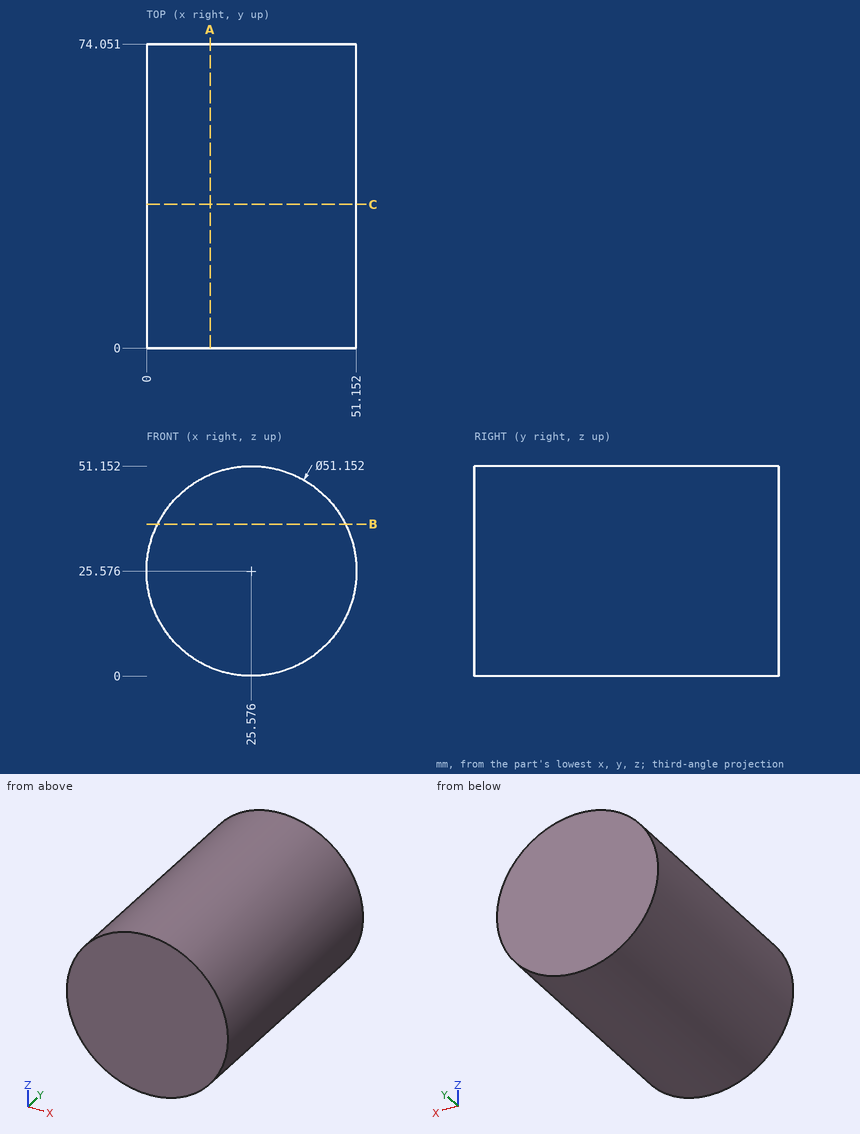
Answer from the drawing. Dimensions are ordinates in mm from the lowest x, y and z of the part. Round coordinates to 2 decimals unless told otherwise and drop trailing zeros. Write each loop counter-clockwise with the first axis right and the second up, starting at its lowest first coordinate (ties: lowest second). Pieces come first, ordered by that corner, then holes.
1. The part is cut by section B-B, the plane z = 37. Determine the outline of the cut face in (x, y), then the cut area to 3 significant figures.
2. The part is cut by section C-C, the plane y = 35. Determine the outline of the cut face in (x, z), then the cut area to 4 significant figures.
3. The part is cut by section A-A, the plane x = 15.5. Determine the outline of the cut face in (y, z).
4. Given pin 1 Ø10 at (y, z) = (12.5, 45.5) entering from +X (1 decimal); pin 2 Ø12 at (x, y) = (17.5, 21) entering from -Z; pin 3 Ø1 at (y, z) = (29.5, 17.5) entering from +X, each flat-ended and moving along its own axis, determine where each tip first touches the part or whether it passes through.
5. Straight lines are drawn through the part: L1, parallel to X at y = 61.5, z = 26; L2, parallel to Z at x = 25, y = 3 (1 decimal). For each, find the intervals that lie inside material, in ascending order.
Values:
1. outline: (2.69, 0) - (48.46, 0) - (48.46, 74.05) - (2.69, 74.05) - close
1. area: 3,390 mm2
2. outline: circle Ø51.15 at (25.58, 25.58)
2. area: 2,055 mm2
3. outline: (0, 2.07) - (74.05, 2.07) - (74.05, 49.08) - (0, 49.08) - close
4. pin 1: stops at x = 46.3
4. pin 2: stops at z = 0.08
4. pin 3: stops at x = 50
5. L1: x = 0 to 51.15
5. L2: z = 0 to 51.1
